The listing builds one solid part. Answer for the finished solid, in the listing's coordinates (mm). A direction names the side the tool comes from. Coordinates: 2 decimals unless noted, no trailing zeros. Loops run counter-clockwise (first coordinate to the right, second up) from the corner with the lowest first, then second, coordinate; pieces in that order, holes last. Notation, with made-up numbers: M 48.5,62 L 85.5,62 A22 cw 85.5,85 Z; hole C 47.25,-4 d9. An arc over 180 degrees is marked long. Answer in a Markdown table with one row per item. Add a question column.
from build123d import *

# Parameters (mm, degrees)
SKETCH1_R           = 1.5
BOSS_EXTRUDE1_DEPTH = 5
BOSS_EXTRUDE2_DEPTH = 1.5
FILLET1_R           = 1


with BuildPart() as part:
    # Sketch1 → Boss-Extrude1 (new body)
    with BuildSketch(Plane.XY):
        with BuildLine():
            Line((-5.112484719, 9.45), (-3.244461456, -0.602884615))
            ThreePointArc((-3.244461456, -0.602884615), (0, -3.3), (3.244461456, -0.602884615))
            Line((3.244461456, -0.602884615), (5.112484719, 9.45))
            ThreePointArc((5.112484719, 9.45), (0, 15.6), (-5.112484719, 9.45))
        make_face()
        Circle(SKETCH1_R, mode=Mode.SUBTRACT)
    extrude(amount=BOSS_EXTRUDE1_DEPTH)

    # Sketch2 → Boss-Extrude2 (add)
    with BuildSketch(Plane.XY.offset(5)):
        with BuildLine():
            Line((-3.017059628, 9.742178321), (3.017059628, 9.742178321))
            ThreePointArc((3.017059628, 9.742178321), (3.724166409, 10.03507154), (4.017059628, 10.742178321))
            Line((4.017059628, 10.742178321), (4.017059628, 11.029697433))
            Line((4.017059628, 11.029697433), (-4.017059628, 11.029697433))
            Line((-4.017059628, 11.029697433), (-4.017059628, 10.742178321))
            ThreePointArc((-4.017059628, 10.742178321), (-3.724166409, 10.03507154), (-3.017059628, 9.742178321))
        make_face()
    extrude(amount=BOSS_EXTRUDE2_DEPTH)

    # Fillet1
    fillet1_edges = [part.edges().sort_by_distance(p)[0] for p in [
        (4.017059628, 10.885937877, 6.5),
        (-4.017059628, 10.885937877, 6.5),
        (-3.724166409, 10.03507154, 6.5),
        (0, 9.742178321, 6.5),
        (3.724166409, 10.03507154, 6.5),
    ]]
    fillet(fillet1_edges, radius=FILLET1_R)


solid = part.part
(1) A cutting plane is placed at B-B (y = 0). Give the vertices of the cut face in (x, z).
(2) A cutting plane is placed at A-A (x = 0). Give the vertices of the cut face in (y, z), plus the area to 3 significant figures.
(3) For faces 4 (the face through (-3.73, 10.04, 5.25)), 5 (the face through (4.165, 4.353, 2.465)), 6 (the face through (3.72, 10.03, 5.25)), 7 (the face through (0, 11.03, 6)), determine the directions among +Z, -Z, +X, -X, +Y, -Y from which every point of the face is accessible in a straight line to the end or side of a thin tool.
(4) The mould has two halves that part along X. Classify faces 1 (the face through (-1.5, 0.07, 2.46)), 2 (the face through (0, 6, 5)), 3 (the face through (-0.1, -3.3, 2.5)): released by +X, released by -X, zero draft, split by the parting line, or undercut.
(5) A cutting plane is placed at C-C (z = 1). Give the vertices of the cut face in (x, y).
(6) Straight lines are drawn through the part: line 1 (Y direction, x = 0, z = 2.85); line 2 (Z direction, x = -3.25, y = 5); line 3 (Y direction, x = 1, z = 3.5). For each, find the intervals that lie inside material, in ascending order.
(7) Each of these flat-tipped pins is pushed along its axis until it touches: pin 1 (3 mm diameter, centred on x = 3.5, y = 6, fed in from -Z); pin 2 (0.8 mm diameter, centred on x = 2, z = 5.5, fed in from +Y); pin 3 (5 mm diameter, centred on x = 0, y = 6, fed in from +Z); pin 4 (2.5 mm diameter, centred on x = 0, y = 0, fed in from -Z). Where does it stop, or does it pass through?
(8) A cutting plane is placed at D-D (x = -3.75). Give the vertices of the cut face in (y, z), plus the area to 3 significant figures.
Solved:
| question | item | result |
|---|---|---|
| 1 | outline | M -3.36,0 L -1.5,0 L -1.5,5 L -3.36,5 Z; M 1.5,0 L 3.36,0 L 3.36,5 L 1.5,5 Z |
| 2 | outline | M -3.3,0 L -1.5,0 L -1.5,5 L -3.3,5 Z; M 1.5,0 L 15.6,0 L 15.6,5 L 11.03,5 L 11.03,6.5 L 10.74,6.5 A1 ccw 9.74,5.5 L 9.74,5 L 1.5,5 Z |
| 2 | area | 81.2 mm² |
| 3 | face 4 | +Z, -X, -Y |
| 3 | face 5 | +Z, -Z, +X, -Y |
| 3 | face 6 | +Z, +X, -Y |
| 3 | face 7 | +Z, +X, -X, +Y |
| 4 | face 1 | undercut |
| 4 | face 2 | zero draft |
| 4 | face 3 | split by the parting line |
| 5 | outline | M -5.11,9.45 L -3.24,-0.6 A3.3 ccw 3.24,-0.6 L 5.11,9.45 A5.2 ccw long Z; hole C 0,0 d3 |
| 6 | line 1 | y = -3.3 to -1.5, 1.5 to 15.6 |
| 6 | line 2 | z = 0 to 5 |
| 6 | line 3 | y = -3.14 to -1.12, 1.12 to 15.5 |
| 7 | pin 1 | stops at z = 0 |
| 7 | pin 2 | stops at y = 11.03 |
| 7 | pin 3 | stops at z = 5 |
| 7 | pin 4 | passes through |
| 8 | outline | M 2.12,0 L 14,0 L 14,5 L 11.03,5 L 11.03,6.18 L 10.74,6.18 A0.68 ccw 10.06,5.5 L 10.06,5 L 2.12,5 Z |
| 8 | area | 60.5 mm² |
